from build123d import *

# Parameters (mm, degrees)
F0_W      = 80
F0_H      = 30
F1_DEPTH  = 10
F2_SIZE   = 9.99999
F4_DEPTH  = 40
F4_FACE_W = 40
F4_FACE_H = 30
F5_DEPTH  = 40


# Not quite as in the source:
# - a fillet or chamfer is up to 0.001 mm smaller than in the source, because OpenCascade refuses the exact size


with BuildPart() as f1:
    # F0 (on Top) → F1 (new body)
    with BuildSketch(Plane.XY):
        Rectangle(F0_W, F0_H)
    extrude(amount=F1_DEPTH)

    # F2 (size 10 in the source; OpenCascade refuses exactly that, so slightly less here)
    f2_edges = [f1.edges().sort_by_distance(p)[0] for p in [
        (40, 0, 10),
        (-40, 0, 10),
    ]]
    chamfer(f2_edges, length=F2_SIZE)

    # F3 (on Top) → F4 (join)
    with BuildSketch(Plane.XY):
        Polygon((20, -15), (20, 15), (16.5369563365, -15), align=None)
        Polygon((16.5369563365, -15), (20, 15), (-16.5369563365, 15), (-20, -15), align=None)
        Polygon((-20, -15), (-16.5369563365, 15), (-20, 15), align=None)
    extrude(amount=F4_DEPTH)

    # F3 (on Top) + F4_face (on face) → F5 (join)
    with BuildSketch(Plane.XY):
        Polygon((20, -15), (20, 15), (16.5369563365, -15), align=None)
        Polygon((16.5369563365, -15), (20, 15), (-16.5369563365, 15), (-20, -15), align=None)
        Polygon((-20, -15), (-16.5369563365, 15), (-20, 15), align=None)
    with BuildSketch(Plane.XY.offset(40)):
        Rectangle(F4_FACE_W, F4_FACE_H)
    extrude(amount=F5_DEPTH)


solid = f1.part
Part model, mm, in its own coordinate system. A direction names the side the tool comes from. Round coordinates to 2 decimals unless told otherwise and drop trailing zeros. Order: outer loops, then holes, each group sorted by start corner. A loop starts at its lowest first (then second) coordinate and runs counter-clockwise, first axis right, second up. Notation, with made-up numbers: (-25, 28.5) -> (-11, 28.5) arc R17 ccw to (-11, 44.5) -> close; hole circle Ø5 at (70, 30). An arc over 180 degrees is marked (long way). Put each result on its own line as item: value.
Q1. Pin check, flat tips, straight feed: pin 1 Ø4 at (y, z) = (-12, 40) entering from +X; pin 2 Ø3 at (x, y) = (-24.5, 3) entering from +Z; pin 3 Ø5 at (y, z) = (0, 33.5) entering from -X; pin 4 Ø5 at (x, y) = (12, -11) entering from -Z. Stop position of each tip, or through.
From the geometry:
pin 1: stops at x = 20
pin 2: stops at z = 10
pin 3: stops at x = -20
pin 4: stops at z = 0
Q2. Tool access for faces 1 (the face through (20, 0, 45)), 2 (the face through (-1, 15, 39)), 3 (the face through (-20, 0, 45)): list every direction of +Z, -Z, +X, -X, +Y, -Y with a clear straight run to the whole face (end or side of a thin tool).
From the geometry:
face 1: +Z, +X, +Y, -Y
face 2: +Z, -Z, +X, -X, +Y
face 3: +Z, -X, +Y, -Y
Q3. Band-saw the part on B-B (x = 22.5). Give the cut face in (y, z), and give its area (3 significant figures).
From the geometry:
outline: (-15, 0) -> (15, 0) -> (15, 10) -> (-15, 10) -> close
area: 300 mm2
Q4. Band-saw the part on C-C (z = 19.5). Give the cut face in (x, y), and give its area (3 significant figures).
From the geometry:
outline: (-20, -15) -> (20, -15) -> (20, 15) -> (-20, 15) -> close
area: 1,200 mm2
Q5. Wall check: line 1 (Z direction, x = 29, y = 2); line 2 (X direction, y = 5.5, z = 61); line 3 (Z direction, x = 35, y = -4). Give the ranges that are in metal, low to high. Write a range as [from, to].
From the geometry:
line 1: z = [0, 10]
line 2: x = [-20, 20]
line 3: z = [0, 5]
